Read the model definition and answer for the solid it produces. Units are mm, in the model's axes. Face numbers are marked on the shaded views. A direction names the side the tool comes from. Coordinates: 2 decimals unless noted, no trailing zeros. Write each loop counter-clockwise with the first axis right and the second up, starting at its lowest first coordinate (ties: lowest second). Pieces come first, ordered by that corner, then holes. Notation, with made-up numbers: M 25,10 L 59,10 A27 ccw 59,29 Z; hole C 53.5,51.25 d10. An arc over 180 degrees is marked long. Use a Markdown table: item, result. Add a question column.
from build123d import *

# Parameters (mm, degrees)
SKETCH1_W           = 18
SKETCH1_H           = 34
SKETCH1_R           = 1.75
BOSS_EXTRUDE1_DEPTH = 19
CUT_EXTRUDE1_DEPTH  = 18
CHAMFER1_SIZE       = 6
CHAMFER2_SIZE       = 2
CHAMFER3_SIZE       = 4
SKETCH3_W           = 10
SKETCH3_H           = 4
CUT_EXTRUDE2_DEPTH  = 2


with BuildPart() as part:
    # Sketch1 → Boss-Extrude1 (new body)
    with BuildSketch(Plane.XY):
        Rectangle(SKETCH1_W, SKETCH1_H)
        with Locations((5.5, 6)):
            Circle(SKETCH1_R, mode=Mode.SUBTRACT)
        with Locations((-5.5, 6)):
            Circle(SKETCH1_R, mode=Mode.SUBTRACT)
    extrude(amount=BOSS_EXTRUDE1_DEPTH)

    # Sketch2 → Cut-Extrude1 (cut)
    with BuildSketch(Plane(origin=(9, 0, 0), x_dir=(0, 0, -1), z_dir=(1, 0, 0))):
        Polygon((-19, 17), (-16, 17), (-16, -10), (-19, -13), align=None)
    extrude(amount=-CUT_EXTRUDE1_DEPTH, mode=Mode.SUBTRACT)

    # Chamfer1
    chamfer1_edges = [part.edges().sort_by_distance(p)[0] for p in [
        (0, 17, 16),
    ]]
    chamfer(chamfer1_edges, length=CHAMFER1_SIZE)

    # Chamfer2
    chamfer2_edges = [part.edges().sort_by_distance(p)[0] for p in [
        (-9, 17, 5),
        (9, 17, 5),
    ]]
    chamfer(chamfer2_edges, length=CHAMFER2_SIZE)

    # Chamfer3
    chamfer3_edges = [part.edges().sort_by_distance(p)[0] for p in [
        (-9, -15, 19),
        (9, -15, 19),
    ]]
    chamfer(chamfer3_edges, length=CHAMFER3_SIZE)

    # Sketch3 → Cut-Extrude2 (cut)
    with BuildSketch(Plane(origin=(0, 17, 0), x_dir=(1, 0, 0), z_dir=(0, 1, 0))):
        with Locations((0, -2)):
            Rectangle(SKETCH3_W, SKETCH3_H)
    extrude(amount=-CUT_EXTRUDE2_DEPTH, mode=Mode.SUBTRACT)


solid = part.part
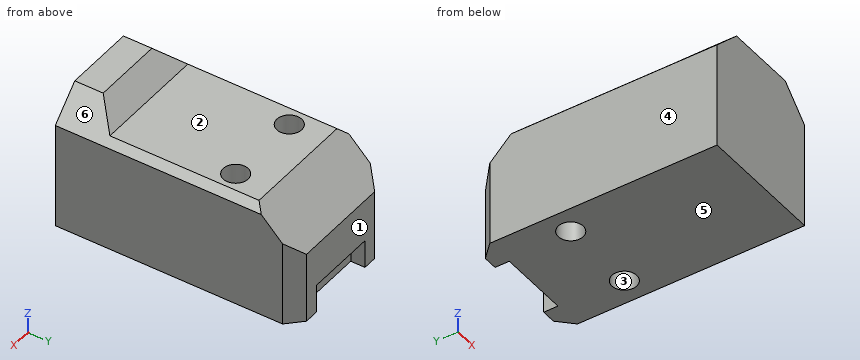
Item 1: Each of these flat-tipped pins is pushed along its axis until it touches: pin 1 (1 mm diameter, centred on y = 16.5, z = 2.5, fed in from +X); pin 2 (2 mm diameter, centred on x = -0.5, z = 1.5, fed in from +Y); pin 3 (3 mm diameter, centred on x = -5.5, y = 6, fed in from -Z); pin 4 (5.5 mm diameter, centred on x = 5.5, y = 6, fed in from +Z). Where does it stop, or does it pass through?
Item 2: Find section B-B on z = 4.5. Give the vertices of the cut face in (x, y).
Item 3: Find section A-A on x = 5.5. Give the vertices of the cut face in (y, z).
Item 4: Find section D-D on y = -3. Give the vertices of the cut face in (x, z).
Item 5: Determine the mould class of the marked faces 3, 4, 5 and 6 for opening direction X: pulls with the +X half, pulls with the -X half, needs draft (parallel to the pull), parting line crosses it, or undercut.
Item 6: Find section C-C on y = 6. Give the vertices of the cut face in (x, z).
Item 7: Consider probe 1 along X at (y, z) = (6, 11.5); probe 2 along Y at (x, z) = (-5.5, 9.25); probe 3 along Z at (x, y) = (-4.5, 8). Determine where each line is inside the solid, lowest interval first.
Item 8: For the marked faces 1 and 2, determine the directions among +Z, -Z, +X, -X, +Y, -Y from which every point of the face is accessible in a straight line to the end or side of a thin tool.
Geometry says:
| question | item | result |
|---|---|---|
| 1 | pin 1 | stops at x = 8 |
| 1 | pin 2 | stops at y = 15 |
| 1 | pin 3 | passes through |
| 1 | pin 4 | stops at z = 16 |
| 2 | outline | M -9,-17 L 9,-17 L 9,15 L 7,17 L -7,17 L -9,15 Z; hole C -5.5,6 d3.5; hole C 5.5,6 d3.5 |
| 3 | outline | M -17,0 L 4.25,0 L 4.25,16 L -10,16 L -12.5,18.5 L -17,18.5 Z; M 7.75,0 L 17,0 L 17,10 L 11,16 L 7.75,16 Z |
| 4 | outline | M -9,0 L 9,0 L 9,15 L 8,16 L -8,16 L -9,15 Z |
| 5 | face 3 | undercut |
| 5 | face 4 | pulls with the -X half |
| 5 | face 5 | needs draft |
| 5 | face 6 | pulls with the +X half |
| 6 | outline | M -9,0 L -7.25,0 L -7.25,16 L -8,16 L -9,15 Z; M -3.75,0 L 3.75,0 L 3.75,16 L -3.75,16 Z; M 7.25,0 L 9,0 L 9,15 L 8,16 L 7.25,16 Z |
| 7 | probe 1 | x = -9 to -7.25, -3.75 to 3.75, 7.25 to 9 |
| 7 | probe 2 | y = -17 to 4.25, 7.75 to 17 |
| 7 | probe 3 | z = 0 to 16 |
| 8 | face 1 | +Z, -Z, +X, -X, +Y |
| 8 | face 2 | +Z, +X, -X, +Y |
